Autodesk Inventor part; units mm, degrees
ref_plane "Work Plane1" through (0, 0, 0) normal (0.7071, 0, -0.7071) x (0, 1, 0)
ref_plane "XZ Plane" through (0, 0, 0) normal (0, 1, 0) x (-1, 0, 0)
ref_plane "XY Plane" through (0, 0, 0) normal (0, 0, 1) x (1, 0, 0)
sketch "Sketch1" plane through (0, 0, 0) normal (0, 0, 1) x (1, 0, 0)
  line L0 (0, 0) -> (0, -20.7931)
  line L1 (117, 0) -> (117, 43)
  line L2 (117, 43) -> (114.25, 43)
  line L3 (114.25, 43) -> (114.25, 3)
  line L4 (114.25, 3) -> (116, 3)
  line L5 (116, 3) -> (116, 0)
  line L6 (116, 0) -> (117, 0)
  dimension "d1" = 234
  dimension "d2" = 228.5
  dimension "d6" = 1
  dimension "d7" = 3
revolve "Revolution1" add sketch "Sketch1" angle 360 about axis through (0, 0, 0) along (0, -1, 0)
ref_plane "Work Plane1" through (0, 0, 0) normal (0.7071, 0, -0.7071) x (0, 1, 0)
sketch "Sketch2" plane through (0, 0, 0) normal (0.7071, 0, -0.7071) x (0, 1, 0)
  circle A0 centre (36.5, 0) radius 2.5
  line L0 (43, 117) -> (43, -117) construction
  point P0 (0, 0)
  point P1 (43, 0)
  dimension "d9" = 5
  dimension "d10" = 6.5
extrude "Extrusion1" cut sketch "Sketch2" along normal through all both and the other way through all
pattern_circular "Circular Pattern1" count 4 over 360 about axis through (0, 21.5, 0) along (0, -1, 0) of "Extrusion1"
properties part number "bucket" material "ABS Plastic"
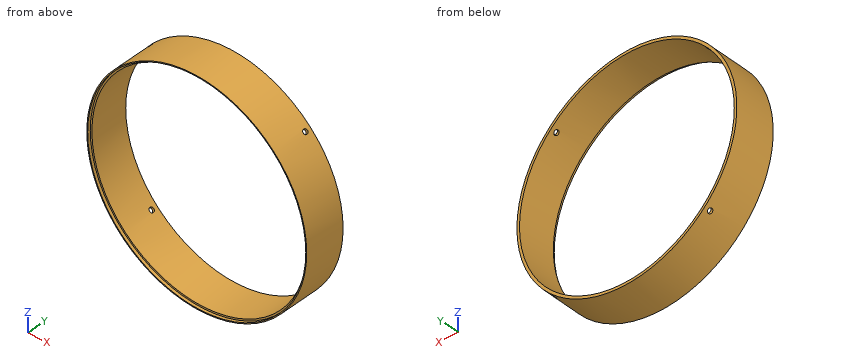
The model under review builds one solid part; all positions refer to its coordinate system, in mm. Round coordinates to 2 decimals unless told otherwise and drop trailing zeros. Order: outer loops, then holes, each group sorted by start corner. A loop starts at its lowest first (then second) coordinate and runs counter-clockwise, first axis right, second up. Notation, with made-up numbers: (-39.5, 41) -> (17.5, 41) arc R8 ccw to (17.5, 55) -> close; hole circle Ø7 at (55, 68). An arc over 180 degrees is marked (long way). One line per item, written item: value. Start each with the question number.
Q1. Wall thickness on line 1 (Z direction, x = 0, y = 0.75); line 2 (Z direction, x = 0, y = 31.5); line 3 (X direction, y = 5.5, z = 47): over which ranges is each line inside the solid? List them lowest first.
Q2. Take a section at C-C (y = 11). Write out the cut boundary in (x, z), and give its area (3 significant figures).
Q3. Take a section at B-B (x = 0). Write out the cut boundary in (y, z), and give its area (3 significant figures).
Q4. Clearance check with flat-ended pins moving along their axes: pin 1 Ø12 at (y, z) = (12, 3.5) entering from -X; pin 2 Ø3 at (x, y) = (61.5, 19) entering from -Z; pin 3 Ø6 at (x, y) = (84.5, 11) entering from +Z; pin 4 Ø1 at (x, y) = (-41.5, 34) entering from -Z. State where each tip first meets the part, or that it passes through.
Q5. Take a section at A-A (z = 0). Write out the cut boundary in (x, y), and give its area (3 significant figures).
Reported:
1. line 1: z = -117 to -116, 116 to 117
1. line 2: z = -117 to -114.25, 114.25 to 117
1. line 3: x = -107.14 to -104.13, 104.13 to 107.14
2. outline: circle Ø234 at (0, 0); hole circle Ø228.5 at (0, 0)
2. area: 2,000 mm2
3. outline: (0, -117) -> (43, -117) -> (43, -114.25) -> (3, -114.25) -> (3, -116) -> (0, -116) -> close; (0, 116) -> (3, 116) -> (3, 114.25) -> (43, 114.25) -> (43, 117) -> (0, 117) -> close
3. area: 226 mm2
4. pin 1: stops at x = -117
4. pin 2: stops at z = -100.44
4. pin 3: stops at z = 83.94
4. pin 4: stops at z = -109.58
5. outline: (-117, 0) -> (-116, 0) -> (-116, 3) -> (-114.25, 3) -> (-114.25, 43) -> (-117, 43) -> close; (114.25, 3) -> (116, 3) -> (116, 0) -> (117, 0) -> (117, 43) -> (114.25, 43) -> close
5. area: 226 mm2
